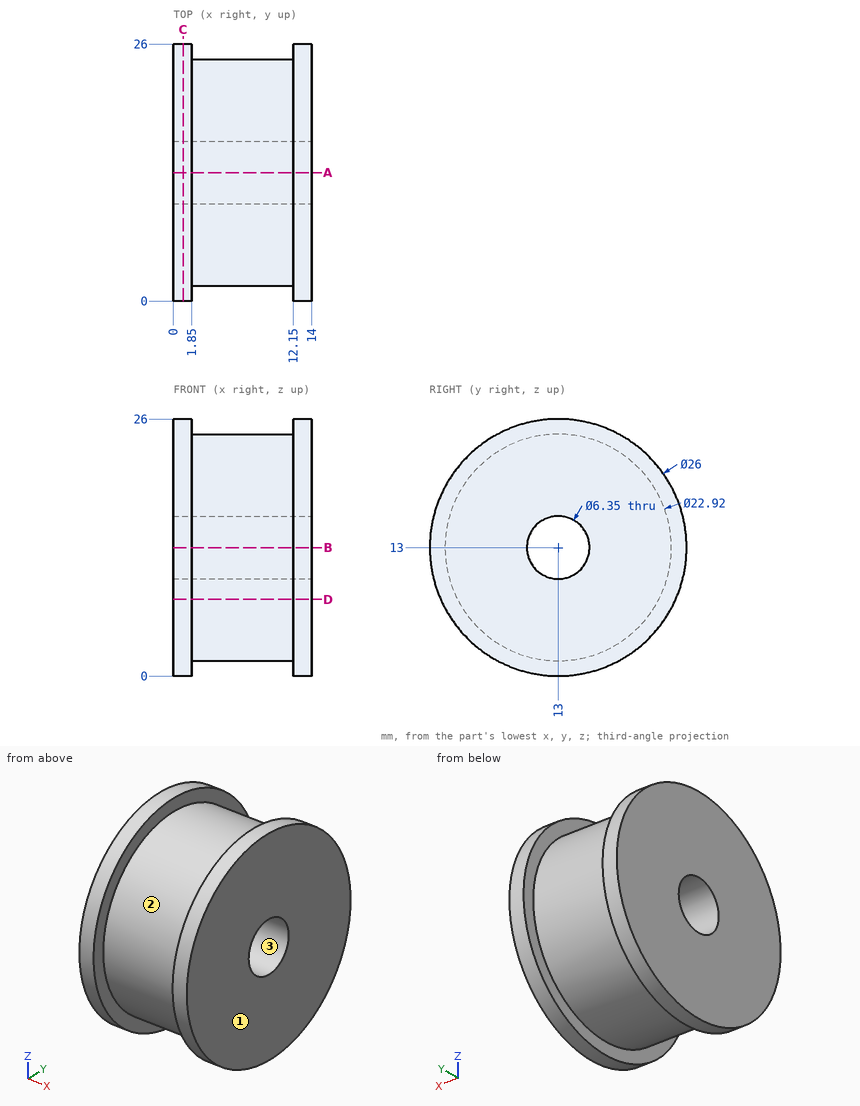
Verification items for this drawing (mm, ordinates from the low corner). Coordinates: 2 decimals unless noted, no trailing zeros. Order: outer loops, then holes, each group sorted by start corner. A loop starts at its lowest first (then second) coordinate and runs counter-clockwise, first axis right, second up. Notation, with made-up numbers: (-25.5, 41.25) - (-19.5, 41.25) arc R24 ccw to (-19.5, 78.25) - close; hole circle Ø7 at (63, 10). An arc over 180 degrees is marked (long way). Answer in a Markdown table with one row per item. Add a question column.
1. Material ranges on L1, parallel to Y at x = 6.5, z = 13 (3 decimals); L2, parallel to Y at x = 1.75, z = 13 (3 decimals); L3, parallel to X at y = 24.75, z = 13.5, recorded low to high. Write a range as [from, to].
2. Section check D-D (z = 7.75). Enter the section's corners in (x, y), plus the area to 3 significant figures.
3. Section check C-C (x = 1). Enter the section's corners in (y, z) (3 decimals), plus the area to 3 significant figures.
4. Section check A-A (y = 13). Enter the section's corners in (x, z) (3 decimals), plus the area to 3 significant figures.
5. Gauge pin test, flat ends, axial feed: pin 1 Ø5 at (x, y) = (4, 16.5) entering from -Z; pin 2 Ø1.5 at (x, y) = (8, 6) entering from +Z; pin 3 Ø6 at (x, z) = (4.5, 8) entering from +Y. Record the tip position at first contact, or that the pin passes through.
6. Draft check along Z on the marked faces 1, 2 and 3. Enter one of: +Z half, -Z half, draft (parallel to the pull), parting line (faces both ways), or undercut.
Data:
| question | item | result |
|---|---|---|
| 1 | L1 | y = [1.54, 9.825], [16.175, 24.46] |
| 1 | L2 | y = [0, 9.825], [16.175, 26] |
| 1 | L3 | x = [0, 1.85], [12.15, 14] |
| 2 | outline | (0, 1.11) - (1.85, 1.11) - (1.85, 2.81) - (12.15, 2.81) - (12.15, 1.11) - (14, 1.11) - (14, 24.89) - (12.15, 24.89) - (12.15, 23.19) - (1.85, 23.19) - (1.85, 24.89) - (0, 24.89) - close |
| 2 | area | 298 mm² |
| 3 | outline | circle Ø26 at (13, 13); hole circle Ø6.35 at (13, 13) |
| 3 | area | 499 mm² |
| 4 | outline | (0, 0) - (1.85, 0) - (1.85, 1.54) - (12.15, 1.54) - (12.15, 0) - (14, 0) - (14, 9.825) - (0, 9.825) - close; (0, 16.175) - (14, 16.175) - (14, 26) - (12.15, 26) - (12.15, 24.46) - (1.85, 24.46) - (1.85, 26) - (0, 26) - close |
| 4 | area | 243 mm² |
| 5 | pin 1 | stops at z = 0.19 |
| 5 | pin 2 | stops at z = 22.61 |
| 5 | pin 3 | stops at y = 25.49 |
| 6 | face 1 | draft |
| 6 | face 2 | parting line |
| 6 | face 3 | undercut |
